```python
from build123d import *

# Parameters (mm, degrees)
SKETCH2_W           = 203.2
SKETCH2_H           = 203.2
BOSS_EXTRUDE1_DEPTH = 6.35
SKETCH3_W           = 22.86
SKETCH3_H           = 24.6
BOSS_EXTRUDE2_DEPTH = 16.51
CUT_EXTRUDE1_START  = -203.2
SKETCH4_W           = 12.508
SKETCH4_H           = 10.508
CUT_EXTRUDE1_DEPTH  = 203.2


with BuildPart() as part:
    # Sketch2 → Boss-Extrude1 (new body)
    with BuildSketch(Plane(origin=(0, 0, 0), x_dir=(1, 0, 0), z_dir=(0, 1, 0))):
        with Locations((101.6, -101.6)):
            Rectangle(SKETCH2_W, SKETCH2_H)
    extrude(amount=BOSS_EXTRUDE1_DEPTH)

    # Sketch3 → Boss-Extrude2 (add)
    with BuildSketch(Plane(origin=(0, 6.35, 0), x_dir=(1, 0, 0), z_dir=(0, 1, 0))):
        with Locations((191.77, -190.9)):
            Rectangle(SKETCH3_W, SKETCH3_H)
        with Locations((11.43, -190.9)):
            Rectangle(SKETCH3_W, SKETCH3_H)
        with Locations((11.43, -12.3)):
            Rectangle(SKETCH3_W, SKETCH3_H)
        with Locations((191.77, -12.3)):
            Rectangle(SKETCH3_W, SKETCH3_H)
    extrude(amount=BOSS_EXTRUDE2_DEPTH)

    # Sketch4 → Cut-Extrude1 (cut)
    with BuildSketch(Plane(origin=(203.2, 0, 0), x_dir=(0, 0, -1), z_dir=(1, 0, 0)).offset(CUT_EXTRUDE1_START)):
        with Locations((-190.85, 11.604)):
            Rectangle(SKETCH4_W, SKETCH4_H)
        with Locations((-12.35, 11.604)):
            Rectangle(SKETCH4_W, SKETCH4_H)
    extrude(amount=CUT_EXTRUDE1_DEPTH, mode=Mode.SUBTRACT)


solid = part.part
```
Geometry: final body of the model. Coordinates: model frame, mm. A direction names the side the tool comes from. Round coordinates to 2 decimals unless told otherwise and drop trailing zeros. Write each loop counter-clockwise with the first axis right and the second up, starting at its lowest first coordinate (ties: lowest second). Pieces come first, ordered by that corner, then holes.
Item 1: Section query C-C (z = 95.5). Return loops of the section in (x, y).
Item 2: Mould query, pull axis Z, two halves, no side actions, for faces 4 (the face through (100, 6, 0)), 5 (the face through (192, 22.86, 12)), 6 (the face through (192, 14, 24.6)). Classes: +Z half, -Z half, draft (parallel to the pull), parting line (faces both ways), or undercut.
Item 3: Pin query (flat end, axial travel): P1, Ø10, axis at x = 129, z = 24, coming from the +Y side; P2, Ø11.5, axis at x = 12.5, y = 11.5, coming from the -Z side. Return the tip coordinate at first contact, or that it passes through.
Item 4: Section query B-B (x = 89). Return loops of the section in (y, z).
Item 5: Material intervals for L1, parallel to Z at x = 189, y = 6.5; L2, parallel to X at y = 11.75, z = 184.5; L3, parallel to Y at x = 164, z = 61, sorted ascending.
Item 6: Set-up query: faces 1 (the face through (11, 12, 18.604)), 2 (the face through (22.86, 18, 191)), 3 (the face through (11, 14, 178.6)). Return all of +Z, -Z, +X, -X, +Y, -Y with unobstructed straight access to the full face (end or side cutting, diameter ignored); none if empty.
Item 7: Section query A-A (y = 14.25). Give the number of separate pieces and of enclosed holes in the cut face, plus the area to 3 significant figures.
Completed:
1. outline: (0, 0) - (203.2, 0) - (203.2, 6.35) - (0, 6.35) - close
2. face 4: -Z half
2. face 5: draft
2. face 6: undercut
3. P1: stops at y = 6.35
3. P2: stops at z = 0
4. outline: (0, 0) - (6.35, 0) - (6.35, 203.2) - (0, 203.2) - close
5. L1: z = 0 to 6.1, 18.6 to 24.6, 178.6 to 184.6, 197.1 to 203.2
5. L2: x = 0 to 22.86, 180.34 to 203.2
5. L3: y = 0 to 6.35
6. face 1: +X, -X
6. face 2: +Z, -Z, +Y
6. face 3: +X, -X, +Y
7. separate pieces: 8
7. enclosed holes: 0
7. area: 1,110 mm2
